Design review of the part built by this model. Coordinates are the model's own, in mm. Face numbers are marked on the shaded views. A direction names the side the tool comes from. Give positions to 0.01 mm unless a question says otherwise; leave off trailing zeros. Write each loop counter-clockwise with the first axis right and the second up, starting at its lowest first coordinate (ties: lowest second). Pieces come first, ordered by that corner, then holes. Notation, with made-up numbers: (-22, 34) -> (12, 34) arc R24 ccw to (12, 47) -> close; hole circle Ø11 at (25.5, 7). An arc over 180 degrees is marked (long way). Return JSON: item names as keys, results as strings. Group by question number.
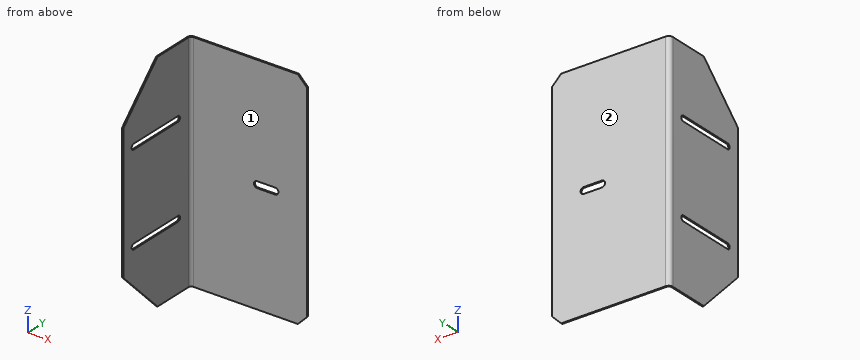
from build123d import *

# Parameters (mm, degrees)
BASE_FLANGE1_DEPTH = 250
CUT_EXTRUDE1_DEPTH = 10
CHAMFER1_SIZE      = 10
CUT_EXTRUDE3_DEPTH = 10
CHAMFER2_SIZE      = 50


# Sheet-metal steps are written as plain solids
with BuildPart() as part:
    # Sketch1 → Base-Flange1 (new body)
    with BuildSketch(Plane.XY):
        with BuildLine():
            Line((0, 0), (0, 95.5))
            ThreePointArc((0, 95.5), (1.318019485, 98.681980515), (4.5, 100))
            Line((4.5, 100), (130, 100))
            Line((130, 100), (130, 98.5))
            Line((130, 98.5), (4.5, 98.5))
            ThreePointArc((4.5, 98.5), (2.378679656, 97.621320344), (1.5, 95.5))
            Line((1.5, 95.5), (1.5, 0))
            Line((1.5, 0), (0, 0))
        make_face()
    extrude(amount=BASE_FLANGE1_DEPTH)

    # Sketch6 → Cut-Extrude1 (cut)
    with BuildSketch(Plane(origin=(0, 100, 0), x_dir=(1, 0, 0), z_dir=(0, 1, 0))):
        with BuildLine():
            Line((95, -128.5), (75, -128.5))
            ThreePointArc((75, -128.5), (71.5, -125), (75, -121.5))
            Line((75, -121.5), (95, -121.5))
            ThreePointArc((95, -121.5), (98.5, -125), (95, -128.5))
        make_face()
    extrude(amount=-CUT_EXTRUDE1_DEPTH, mode=Mode.SUBTRACT)

    # Chamfer1
    chamfer1_edges = [part.edges().sort_by_distance(p)[0] for p in [
        (130, 99.25, 250),
        (130, 99.25, 0),
    ]]
    chamfer(chamfer1_edges, length=CHAMFER1_SIZE)

    # Sketch9 → Cut-Extrude3 (cut)
    with BuildSketch(Plane(origin=(1.5, 0, 0), x_dir=(0, 0, -1), z_dir=(1, 0, 0))):
        with BuildLine():
            Line((-178, 15), (-178, 80))
            ThreePointArc((-178, 80), (-175, 83), (-172, 80))
            Line((-172, 80), (-172, 15))
            ThreePointArc((-172, 15), (-175, 12), (-178, 15))
        make_face()
        with BuildLine():
            Line((-78, 15), (-78, 80))
            ThreePointArc((-78, 80), (-75, 83), (-72, 80))
            Line((-72, 80), (-72, 15))
            ThreePointArc((-72, 15), (-75, 12), (-78, 15))
        make_face()
    extrude(amount=-CUT_EXTRUDE3_DEPTH, mode=Mode.SUBTRACT)

    # Chamfer2
    chamfer2_edges = [part.edges().sort_by_distance(p)[0] for p in [
        (0.75, 0, 250),
        (0.75, 0, 0),
    ]]
    chamfer(chamfer2_edges, length=CHAMFER2_SIZE)


solid = part.part
Q1. For L1, parallel to X at y = 66, z = 112.5; L2, parallel to Y at x = 42, z = 231, list the stretches that pass through material, from the lowest coordinate up. Write a range as from..to.
Q2. Insertion check: pin 1 (0.8 mm diameter, centred on x = 0.5, y = 39, fed in from +Z); pin 2 (1.5 mm diameter, centred on y = 13.5, z = 46, fed in from -X); pin 3 (2 mm diameter, centred on x = 63, z = 161, fed in from -Y). Each pin has a flat end and moves straight along its axis. Give the tip position at first contact, or say it passes through.
Q3. Take a section at D-D, the plane z = 34.5. Give the boundary of the cut face in (x, y).
Q4. Tool access review of the marked faces 1 and 2: name each direction out of +Z, -Z, +X, -X, +Y, -Y from which nothing blocks a thin tool from reaching the whole face with its end or side.
Q5. Take a section at B-B, the plane y = 64. Give the boundary of the cut face in (x, z).
Q6. Take a section at C-C, the plane z = 125. Give the boundary of the cut face in (x, y), plus the area to 3 significant figures.
Q7. Take a section at A-A, the plane x = 88. Give the boundary of the cut face in (y, z), plus the area to 4 significant figures.
Final values:
{
 "1": {"L1": "x = 0..1.5", "L2": "y = 98.5..100"},
 "2": {"pin 1": "stops at z = 239.4", "pin 2": "stops at x = 0", "pin 3": "stops at y = 98.5"},
 "3": {"outline": "(0, 15.5) -> (1.5, 15.5) -> (1.5, 95.5) arc R3 cw to (4.5, 98.5) -> (130, 98.5) -> (130, 100) -> (4.5, 100) arc R4.5 ccw to (0, 95.5) -> close"},
 "4": {"face 1": "+Z, -Z, +X, -Y", "face 2": "+Z, -Z, +X, -X, +Y"},
 "5": {"outline": "(0, 0) -> (1.5, 0) -> (1.5, 72) -> (0, 72) -> close; (0, 78) -> (1.5, 78) -> (1.5, 172) -> (0, 172) -> close; (0, 178) -> (1.5, 178) -> (1.5, 250) -> (0, 250) -> close"},
 "6": {"outline": "(0, 0) -> (1.5, 0) -> (1.5, 95.5) arc R3 cw to (4.5, 98.5) -> (71.5, 98.5) -> (71.5, 100) -> (4.5, 100) arc R4.5 ccw to (0, 95.5) -> close; (98.5, 98.5) -> (130, 98.5) -> (130, 100) -> (98.5, 100) -> close", "area": "300 mm²"},
 "7": {"outline": "(98.5, 0) -> (100, 0) -> (100, 121.5) -> (98.5, 121.5) -> close; (98.5, 128.5) -> (100, 128.5) -> (100, 250) -> (98.5, 250) -> close", "area": "364.5 mm²"}
}
